Read the model definition and answer for the solid it produces. Units are mm, in the model's axes. Face numbers are marked on the shaded views. Give positions to 0.01 mm unless a question says otherwise; leave off trailing zeros. Order: outer loops, then holes, each group sorted by start corner. A loop starts at its lowest first (then second) coordinate and runs counter-clockwise, first axis right, second up.
Autodesk Inventor part; units mm, degrees
ref_plane "YZ Plane" through (0, 0, 0) normal (1, 0, 0) x (0, 1, 0)
ref_plane "XZ Plane" through (0, 0, 0) normal (0, 1, 0) x (-1, 0, 0)
ref_plane "XY Plane" through (0, 0, 0) normal (0, 0, 1) x (1, 0, 0)
sketch "Sketch1" plane through (0, 0, 0) normal (0, 1, 0) x (-1, 0, 0)
  line L0 (0, 0) -> (40, 0)
  line L1 (40, 0) -> (40, -70)
  line L2 (40, -70) -> (0, -70)
  line L3 (0, -70) -> (0, 0)
  circle A0 centre (20, -50) radius 6
  circle A1 centre (20, -20) radius 6
  dimension "d0" = 40
  dimension "d1" = 70
  dimension "d2" = 12
  dimension "d3" = 12
  dimension "d4" = 20
  dimension "d5" = 30
extrude "Extrusion1" add sketch "Sketch1" along normal blind 25.4
fillet "Fillet1" radius 12.7 4 edges at (0, 12.7, -70) (-40, 12.7, -70) (0, 12.7, 0) (-40, 12.7, 0)
properties part number "travel_mount"
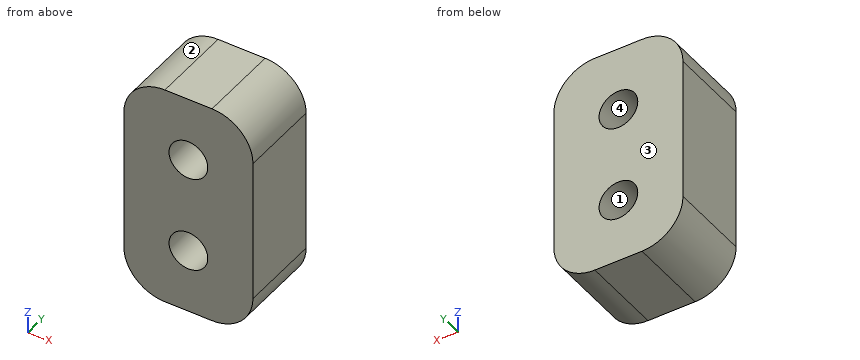
1) For a pull along Z with two mould halves and no side action, classify the marked faces 1, 2, 3 and 4 as released by +Z, released by -Z, zero draft, split by the parting line, or undercut.
Final values:
face 1: undercut
face 2: released by +Z
face 3: zero draft
face 4: undercut
2) The part is cut by section A-A on y = 9. Determine the outline of the cut face in (x, z), and give its area (3 significant figures).
Final values:
outline: (-40, -57.3) arc R12.7 ccw to (-27.3, -70) - (-12.7, -70) arc R12.7 ccw to (0, -57.3) - (0, -12.7) arc R12.7 ccw to (-12.7, 0) - (-27.3, 0) arc R12.7 ccw to (-40, -12.7) - close; hole circle Ø12 at (-20, -50); hole circle Ø12 at (-20, -20)
area: 2,440 mm2
3) The part is cut by section C-C on x = -20. Determine the outline of the cut face in (y, z), and give its area (3 significant figures).
Final values:
outline: (0, -70) - (25.4, -70) - (25.4, -56) - (0, -56) - close; (0, -44) - (25.4, -44) - (25.4, -26) - (0, -26) - close; (0, -14) - (25.4, -14) - (25.4, 0) - (0, 0) - close
area: 1,170 mm2
4) The part is cut by section D-D on z = -49. Determine the outline of the cut face in (x, y).
Final values:
outline: (-40, 0) - (-25.92, 0) - (-25.92, 25.4) - (-40, 25.4) - close; (-14.08, 0) - (0, 0) - (0, 25.4) - (-14.08, 25.4) - close
5) Consider L1, parallel to Z at x = -20, y = 12.5; L2, parallel to Z at x = -24, y = 9; L3, parallel to X at y = 13.75, z = -16.5. Determine where each line is inside the solid, lowest interval first.
Final values:
L1: z = -70 to -56, -44 to -26, -14 to 0
L2: z = -70 to -54.47, -45.53 to -24.47, -15.53 to 0
L3: x = -40 to -24.87, -15.13 to 0
6) The part is cut by section B-B on z = -20. Determine the outline of the cut face in (x, y), and give its area (3 significant figures).
Final values:
outline: (-40, 0) - (-26, 0) - (-26, 25.4) - (-40, 25.4) - close; (-14, 0) - (0, 0) - (0, 25.4) - (-14, 25.4) - close
area: 711 mm2
7) Given pin 1 (5 mm diameter, centred on x = -32.5, y = 9, fed in from +Z); pin 2 (11 mm diameter, centred on x = -20, z = -50, fed in from +Y); pin 3 (5 mm diameter, centred on y = 8, z = -7, fed in from +X); pin 4 (1.5 mm diameter, centred on x = -8, y = 11, fed in from -Z), each flat-ended and moving along its own axis, determine where each tip first touches the part or whether it passes through.
Final values:
pin 1: stops at z = -0.29
pin 2: passes through
pin 3: stops at x = -0.41
pin 4: stops at z = -69.37
